Input: dimensioned drawing with shaded views. Units: mm. Origin: part minimum x, y, z. Give positions to 0.01 mm unless a question says otherwise; leave off trailing zeros. Loops run counter-clockwise (first coordinate to the right, second up) from the corner with the lowest first, then second, coordinate; pieces in that order, holes last. Notation, with made-up numbers: (-10.75, 50.5) -> (4.25, 50.5) arc R20 ccw to (4.25, 86.5) -> close; hole circle Ø5 at (46.25, 4). An arc over 180 degrees is marked (long way). Answer in a Markdown table with one row per item. Add a question column.
1) Section query C-C (y = 68). Return the cut outline in (x, z), plus the area to 3 significant figures.
2) Line query: line 1 (Y direction, x = 82.5, z = 19); line 2 (Z direction, x = 29.5, y = 88); line 3 (Y direction, x = 5, z = 4). Output: solid intervals per line, ascending. Write a range as from..to.
3) First-contact query: P1, Ø10, axis at x = 11.5, y = 59.5, coming from the +Z side; P2, Ø1, axis at x = 77.5, z = 46, coming from the +Y side. Flat tips, straight axial feed; report the tip coordinate or a pass-through.
4) Section query A-A (x = 77.5). Return the cut outline in (y, z).
5) Section query B-B (z = 49.5). Return the cut outline in (x, y), plus the area to 3 significant figures.
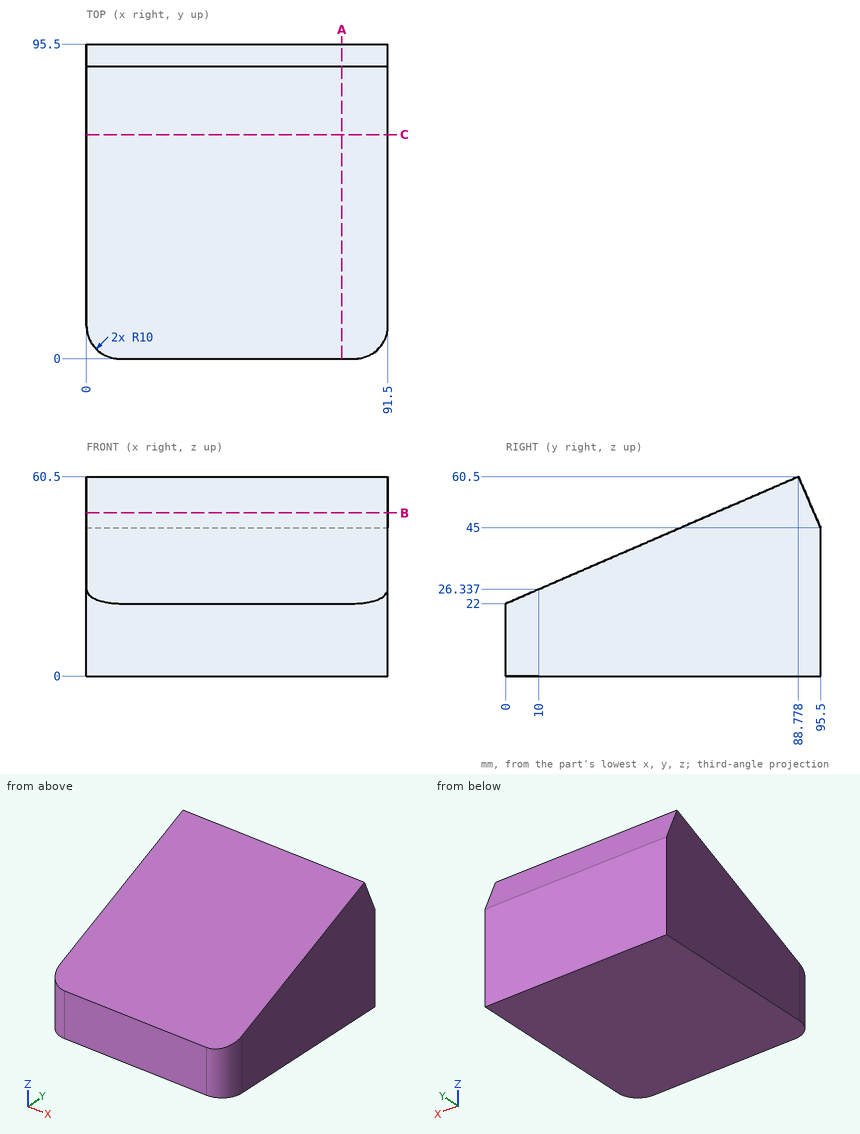
Evaluation:
| question | item | result |
|---|---|---|
| 1 | outline | (0, 0) -> (91.5, 0) -> (91.5, 51.49) -> (0, 51.49) -> close |
| 1 | area | 4,710 mm² |
| 2 | line 1 | 0.05..95.5 |
| 2 | line 2 | 0..60.16 |
| 2 | line 3 | 1.34..95.5 |
| 3 | P1 | z = 49.97 |
| 3 | P2 | y = 95.28 |
| 4 | outline | (0, 0) -> (95.5, 0) -> (95.5, 45) -> (88.78, 60.5) -> (0, 22) -> close |
| 5 | outline | (0, 63.41) -> (91.5, 63.41) -> (91.5, 93.55) -> (0, 93.55) -> close |
| 5 | area | 2,760 mm² |
